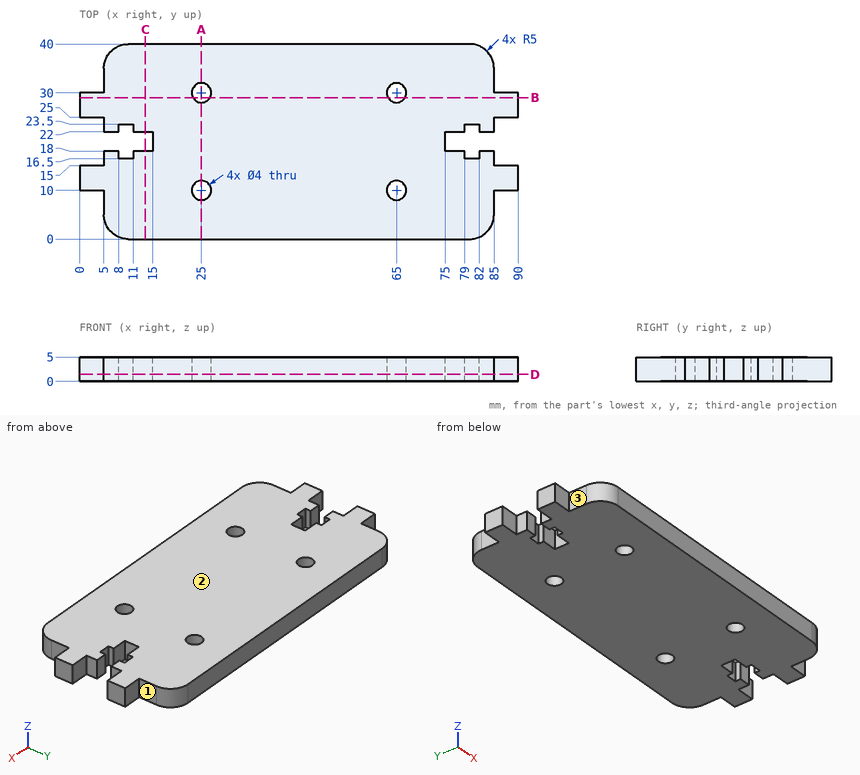
The figure shows three views and two pictorial views of one solid part (mm, origin at its lowest corner). Answer the questions. A direction names the side the tool comes from. Coordinates: 2 decimals unless noted, no trailing zeros. Loops run counter-clockwise (first coordinate to the right, second up) from the corner with the lowest first, then second, coordinate; pieces in that order, holes last. Notation, with made-up numbers: (69.25, 48.5) - (125.25, 48.5) arc R20 cw to (125.25, 61.5) - close; hole circle Ø9 at (66.5, 4). An arc over 180 degrees is marked (long way). Use a Markdown table: item, result. Add a question column.
1) The part is cut by section D-D, the plane z = 1.45. State how many separate pieces and enclosed holes the cut face has, and give its area (3 significant figures).
2) Given pin 1 (0.8 mm diameter, centred on y = 22.5, z = 2.5, fed in from -X); pin 2 (1.5 mm diameter, centred on x = 9, z = 3, fed in from -Y); pin 3 (2.5 mm diameter, centred on x = 7, z = 3.5, fed in from +Y); pin 4 (3.5 mm diameter, centred on x = 65, y = 30, fed in from -Z), each flat-ended and moving along its own axis, determine where each tip first touches the part or whether it passes through.
3) For the marked faces 1, 2 and 3, determine the directions among +Z, -Z, +X, -X, +Y, -Y from which every point of the face is accessible in a straight line to the end or side of a thin tool.
4) The part is cut by section C-C, the plane x = 13.5. Give the vertices of the cut face in (y, z).
5) The part is cut by section B-B, the plane y = 29. Give the vertices of the cut face in (x, z), and give its area (3 significant figures).
6) Find the intervals of material crossed by line 1 (Y direction, x = 25, z = 1.6); line 2 (X direction, y = 23, z = 2.15); line 3 (Y direction, x = 24, z = 1.35), in increasing order.
7) The part is cut by section A-A, the plane x = 25. Give the vertices of the cut face in (y, z).
Here are the results:
| question | item | result |
|---|---|---|
| 1 | separate pieces | 1 |
| 1 | enclosed holes | 4 |
| 1 | area | 3,130 mm^2 |
| 2 | pin 1 | stops at x = 5 |
| 2 | pin 2 | stops at y = 0.01 |
| 2 | pin 3 | stops at y = 39.68 |
| 2 | pin 4 | passes through |
| 3 | face 1 | +Z, -Z, +X, +Y |
| 3 | face 2 | +Z, +X, -X, +Y, -Y |
| 3 | face 3 | +Z, -Z, -X, -Y |
| 4 | outline | (0, 0) - (18, 0) - (18, 5) - (0, 5) - close; (22, 0) - (40, 0) - (40, 5) - (22, 5) - close |
| 5 | outline | (0, 0) - (23.27, 0) - (23.27, 5) - (0, 5) - close; (26.73, 0) - (63.27, 0) - (63.27, 5) - (26.73, 5) - close; (66.73, 0) - (90, 0) - (90, 5) - (66.73, 5) - close |
| 5 | area | 415 mm^2 |
| 6 | line 1 | y = 0 to 8, 12 to 28, 32 to 40 |
| 6 | line 2 | x = 5 to 8, 11 to 79, 82 to 85 |
| 6 | line 3 | y = 0 to 8.27, 11.73 to 28.27, 31.73 to 40 |
| 7 | outline | (0, 0) - (8, 0) - (8, 5) - (0, 5) - close; (12, 0) - (28, 0) - (28, 5) - (12, 5) - close; (32, 0) - (40, 0) - (40, 5) - (32, 5) - close |
